Check sheet for the modelled part. Datum: model origin and axes. Units: mm. Round coordinates to 2 decimals unless told otherwise and drop trailing zeros. Order: outer loops, then holes, each group sorted by start corner. A loop starts at its lowest first (then second) coordinate and runs counter-clockwise, first axis right, second up. Notation, with made-up numbers: (-8, 36) -> (25, 36) arc R26 ccw to (25, 67) -> close; hole circle Ø11 at (36, -20). An arc over 180 degrees is marked (long way). Answer in a Markdown table with one row per item.
from build123d import *

# Parameters (mm, degrees)
SKETCH1_R           = 100
BOSS_EXTRUDE1_DEPTH = 10
SKETCH3_R           = 12.5
CUT_EXTRUDE2_DEPTH  = 20
SKETCH2_R           = 7.5
CUT_EXTRUDE3_DEPTH  = 10
SKETCH5_R           = 15
CUT_EXTRUDE5_DEPTH  = 10
BOSS_EXTRUDE2_START = -10
SKETCH6_R           = 15
BOSS_EXTRUDE2_DEPTH = 10
SKETCH7_R           = 15
CUT_EXTRUDE6_DEPTH  = 30


with BuildPart() as part:
    # Sketch1 → Boss-Extrude1 (new body)
    with BuildSketch(Plane.XY):
        Circle(SKETCH1_R)
    extrude(amount=BOSS_EXTRUDE1_DEPTH)

    # Sketch3 → Cut-Extrude2 (cut)
    with BuildSketch(Plane(origin=(0, 0, 0), x_dir=(-1, 0, 0), z_dir=(0, 0, -1))):
        Circle(SKETCH3_R)
    extrude(amount=-CUT_EXTRUDE2_DEPTH, mode=Mode.SUBTRACT)

    # Sketch2 → Cut-Extrude3 (cut)
    with BuildSketch(Plane.XY.offset(10)):
        with Locations((-75.027755171, 0)):
            Circle(SKETCH2_R)
    extrude(amount=-CUT_EXTRUDE3_DEPTH, mode=Mode.SUBTRACT)

    # Sketch5 → Cut-Extrude5 (cut)
    with BuildSketch(Plane.XY.offset(10)):
        with Locations((34.061352159, 0)):
            Circle(SKETCH5_R)
        with Locations((79.061352159, 0)):
            Circle(SKETCH5_R)
    extrude(amount=-CUT_EXTRUDE5_DEPTH, mode=Mode.SUBTRACT)

    # Sketch6 → Boss-Extrude2 (add)
    with BuildSketch(Plane(origin=(0, 0, 0), x_dir=(-1, 0, 0), z_dir=(0, 0, -1)).offset(BOSS_EXTRUDE2_START)):
        with Locations((-79.061352159, 0)):
            Circle(SKETCH6_R)
    extrude(amount=BOSS_EXTRUDE2_DEPTH)

    # Sketch7 → Cut-Extrude6 (cut)
    with BuildSketch(Plane(origin=(0, 0, 0), x_dir=(-1, 0, 0), z_dir=(0, 0, -1))):
        with Locations((-34.061352159, 60)):
            Circle(SKETCH7_R)
    extrude(amount=-CUT_EXTRUDE6_DEPTH, mode=Mode.SUBTRACT)


solid = part.part
Item 1: Mould release check, pull along X, two halves, no side actions. Record for faces 1 (the cylindrical face through (27.14, 46.692, 4.93)), 2 (the flat face through (-1, -21, 0)), 3 (the cylindrical face through (95.38, 30.04, 4.93)): pulls with the +X half, pulls with the -X half, needs draft (parallel to the pull), parting line crosses it, or undercut.
Result sheet:
| item | result |
|---|---|
| face 1 | undercut |
| face 2 | needs draft |
| face 3 | parting line crosses it |
Item 2: Cross-section at A-A (y = 0). Record the boundary of the cut face in (x, z).
Result sheet:
| item | result |
|---|---|
| outline | (-100, 0) -> (-82.53, 0) -> (-82.53, 10) -> (-100, 10) -> close; (-67.53, 0) -> (-12.5, 0) -> (-12.5, 10) -> (-67.53, 10) -> close; (12.5, 0) -> (19.06, 0) -> (19.06, 10) -> (12.5, 10) -> close; (49.06, 0) -> (100, 0) -> (100, 10) -> (49.06, 10) -> close |
Item 3: Scan lines: line 1 (Y direction, x = 0, z = 6.75); line 2 (X direction, y = -8, z = 3.5); line 3 (Y direction, x = 30, z = 9.75). Record each from-to range of solid material in increasing order. Write a range as [from, to].
Result sheet:
| item | result |
|---|---|
| line 1 | y = [-100, -12.5], [12.5, 100] |
| line 2 | x = [-99.68, -9.6], [9.6, 21.37], [46.75, 99.68] |
| line 3 | y = [-95.39, -14.44], [14.44, 45.56], [74.44, 95.39] |
Item 4: Cross-section at B-B (y = 60). Record the boundary of the cut face in (x, z), and give its area (3 significant figures).
Result sheet:
| item | result |
|---|---|
| outline | (-80, 0) -> (19.06, 0) -> (19.06, 10) -> (-80, 10) -> close; (49.06, 0) -> (80, 0) -> (80, 10) -> (49.06, 10) -> close |
| area | 1,300 mm^2 |
Item 5: Cross-section at D-D (z = 8). Record the boundary of the cut face in (x, y), and give its area (3 significant figures).
Result sheet:
| item | result |
|---|---|
| outline | circle Ø200 at (0, 0); hole circle Ø15 at (-75.03, 0); hole circle Ø25 at (0, 0); hole circle Ø30 at (34.06, 0); hole circle Ø30 at (34.06, 60) |
| area | 29,300 mm^2 |
Item 6: Depth check by flat-ended pin: P1, Ø19.5, axis at x = -75.03, y = 0, coming from the -Z side; P2, Ø4, axis at x = 46.5, z = 1.5, coming from the +Y side; P3, Ø6, axis at x = -69.5, z = 1.5, coming from the -Y side. Enter the tip coordinate at first touch or a pass-through.
Result sheet:
| item | result |
|---|---|
| P1 | stops at z = 0 |
| P2 | stops at y = 89.55 |
| P3 | stops at y = -74.68 |
Item 7: Cross-section at C-C (x = 0). Record the boundary of the cut face in (y, z).
Result sheet:
| item | result |
|---|---|
| outline | (-100, 0) -> (-12.5, 0) -> (-12.5, 10) -> (-100, 10) -> close; (12.5, 0) -> (100, 0) -> (100, 10) -> (12.5, 10) -> close |
